Here's the drawing with two shaded views (mm, measured from the low corner). I have some questions. A direction names the side the tool comes from. Coordinates: 2 decimals unless noted, no trailing zeros. Write each loop counter-clockwise with the first axis right and the second up, starting at its lowest first coordinate (ties: lowest second). Pieces come first, ordered by that corner, then holes. Notation, with made-up numbers: (-20.5, -5.5) - (24.5, -5.5) arc R20 cw to (24.5, 17.5) - close; hole circle Ø9 at (10, 24). An arc over 180 degrees is marked (long way). Answer in a Markdown table with one row per item. Add a question column.
Item 1: We'd pull the mould along X, two halves only. Please class the marked faces 1, 2 and 3: +X half, -X half, draft (parallel to the pull), parting line (faces both ways), or undercut.
Item 2: Imagine slicing it at B-B (y = 17.5). Please give me the cut outline in (x, z).
Item 3: Imagine slicing it at D-D (z = 20.5). Please give me the cut outline in (x, y), plus the area to 3 significant figures.
Item 4: Which directions (+Z, -Z, +X, -X, +Y, -Y) give clear straight access to the entire face, cutting with the end or side of a thin tool? Please do the marked faces 4 and 5.
Item 5: If I drill on probe 1 along Z at (x, y) = (19, 17.75); probe 2 along X at (y, z) = (5, 4); probe 3 along X at (y, z) = (4, 2), over which ranges is the centre line in solid material (lowest first)? Write a range as from..to.
Item 6: Imagine slicing it at A-A (z = 4). Please give me the cut outline in (x, y).
Item 7: I'm going to push flat-ended pins straight in: pin 1 (5 mm diameter, centred on y = 16.5, z = 3, fed in from -X); pin 2 (3 mm diameter, centred on y = 7.5, z = 4, fed in from +X); pin 3 (1 mm diameter, centred on y = 5.5, z = 9.5, fed in from -X). Where does each tip first touch, or does it pass through?
Item 8: Imagine slicing it at C-C (x = 5). Please give me the cut outline in (y, z).
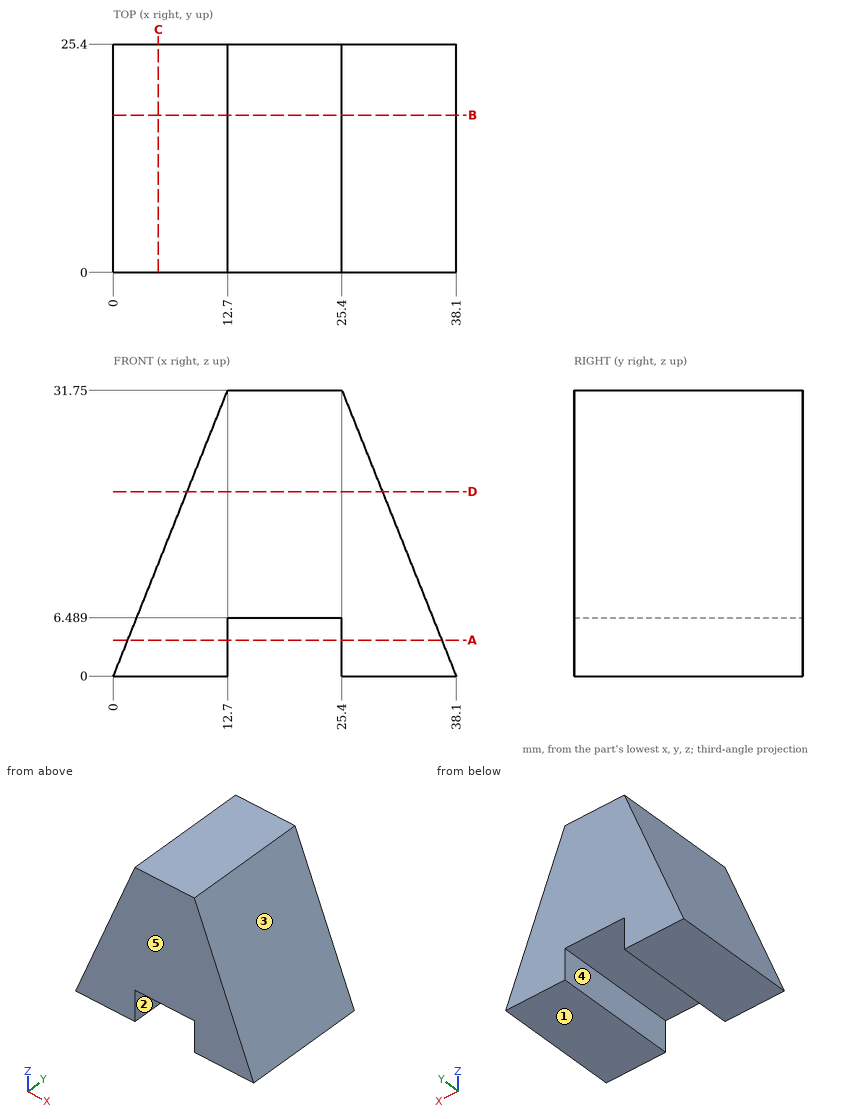
Here are the results:
| question | item | result |
|---|---|---|
| 1 | face 1 | draft |
| 1 | face 2 | undercut |
| 1 | face 3 | +X half |
| 2 | outline | (0, 0) - (12.7, 0) - (12.7, 6.49) - (25.4, 6.49) - (25.4, 0) - (38.1, 0) - (25.4, 31.75) - (12.7, 31.75) - close |
| 3 | outline | (8.2, 0) - (29.9, 0) - (29.9, 25.4) - (8.2, 25.4) - close |
| 3 | area | 551 mm2 |
| 4 | face 4 | -Z, +Y, -Y |
| 4 | face 5 | +Z, -Z, +X, -X, -Y |
| 5 | probe 1 | z = 6.49..31.75 |
| 5 | probe 2 | x = 1.6..12.7, 25.4..36.5 |
| 5 | probe 3 | x = 0.8..12.7, 25.4..37.3 |
| 6 | outline | (1.6, 0) - (12.7, 0) - (12.7, 25.4) - (1.6, 25.4) - close; (25.4, 0) - (36.5, 0) - (36.5, 25.4) - (25.4, 25.4) - close |
| 7 | pin 1 | stops at x = 0.2 |
| 7 | pin 2 | stops at x = 37.1 |
| 7 | pin 3 | stops at x = 3.6 |
| 8 | outline | (0, 0) - (25.4, 0) - (25.4, 12.5) - (0, 12.5) - close |
